For this review, take the finished solid that the model builds, in its own axes (mm). Coordinates: 2 decimals unless noted, no trailing zeros. Loops run counter-clockwise (first coordinate to the right, second up) from the corner with the lowest first, then second, coordinate; pieces in that order, holes last. Notation, with made-up numbers: (-15, -38.75) - (30, -38.75) arc R14 ccw to (30, -12.75) - close; hole circle Ø4 at (22.25, 3.25). An arc over 180 degrees is marked (long way). Use one line per item in the form item = value. Start each with the question number.
1. To check wall thickness, follow probe 1 along Y at (x, z) = (73.25, -4.5); probe 2 along Z at (x, y) = (-114, 27.5); probe 3 along Y at (x, z) = (-128.5, -1.75). State the ranges of each line that lie inside material, in increasing order.
2. Add section C-C on y = 38.5. Give the boundary of the cut face in (x, z), and give its area (3 significant figures).
3. Add section A-A on z = -1.5. Give the boundary of the cut face in (x, y), and give its area (3 significant figures).
4. Add section B-B on x = 83.5. Give the boundary of the cut face in (y, z), and give its area (3 significant figures).
5. Add section D-D on x = -32. Give the boundary of the cut face in (y, z).
6. For pin 1 Ø0.9 at (x, y) = (-120.5, -49) entering from +Z; pin 2 Ø3 at (x, z) = (-115.5, -0.5) entering from -Y; pin 3 Ø3 at (y, z) = (68.08, -4.5) entering from -X; pin 4 Ø4 at (x, z) = (-121.5, -3) entering from -Y, all flat-tipped, find the tip position at first contact; note any pin that passes through.
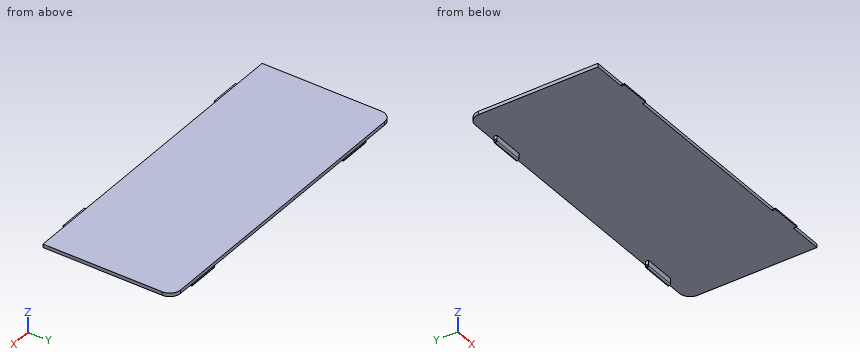
```python
from build123d import *

# Parameters (mm, degrees)
EXTRUDE_1_DEPTH     = 3.2
SKETCH_2_W          = 28
SKETCH_2_H          = 3
CUT_EXTRUDE_1_DEPTH = 2
SKETCH_3_W          = 29
SKETCH_3_H          = 2.8
EXTRUDE_2_DEPTH     = 6.5
SKETCH_4_R          = 1
CUT_EXTRUDE_2_DEPTH = 270.771576627
FILLET_1_R          = 1.5


with BuildPart() as part:
    # 草图1 → 凸台-拉伸1 (new body)
    with BuildSketch(Plane.XY):
        with BuildLine():
            Line((-107.202531646, -47.623114492), (64.797468354, -47.623114492))
            Line((64.797468354, -47.623114492), (64.797468354, -50.623114492))
            Line((64.797468354, -50.623114492), (92.797468354, -50.623114492))
            Line((92.797468354, -50.623114492), (92.797468354, -47.623114492))
            Line((92.797468354, -47.623114492), (123.797468354, -47.623114492))
            Line((123.797468354, -47.623114492), (123.797468354, 62.376885508))
            ThreePointArc((123.797468354, 62.376885508), (120.868536166, 69.447953319), (113.797468354, 72.376885508))
            Line((113.797468354, 72.376885508), (-156.202531646, 72.376885508))
            ThreePointArc((-156.202531646, 72.376885508), (-163.273599457, 69.447953319), (-166.202531646, 62.376885508))
            Line((-166.202531646, 62.376885508), (-166.202531646, -47.623114492))
            Line((-166.202531646, -47.623114492), (-135.202531646, -47.623114492))
            Line((-135.202531646, -47.623114492), (-135.202531646, -50.623114492))
            Line((-135.202531646, -50.623114492), (-107.202531646, -50.623114492))
            Line((-107.202531646, -50.623114492), (-107.202531646, -47.623114492))
        make_face()
    extrude(amount=EXTRUDE_1_DEPTH)

    # 草图2 → 切除-拉伸1 (cut)
    with BuildSketch(Plane.XY.offset(3.2)):
        with Locations((-121.202531646, -49.123114492)):
            Rectangle(SKETCH_2_W, SKETCH_2_H)
        with Locations((78.797468354, -49.123114492)):
            Rectangle(SKETCH_2_W, SKETCH_2_H)
    extrude(amount=-CUT_EXTRUDE_1_DEPTH, mode=Mode.SUBTRACT)

    # 草图3 → 凸台-拉伸2 (add)
    with BuildSketch(Plane.XY):
        with Locations((-121.502531646, 67.976885508)):
            Rectangle(SKETCH_3_W, SKETCH_3_H)
        with Locations((79.097468354, 67.976885508)):
            Rectangle(SKETCH_3_W, SKETCH_3_H)
    extrude(amount=-EXTRUDE_2_DEPTH)

    # 草图4 → 切除-拉伸2 (cut, through all)
    with BuildSketch(Plane(origin=(93.597468354, 0, 0), x_dir=(0, 0, -1), z_dir=(1, 0, 0))):
        with Locations((4.5, 68.076885508)):
            Circle(SKETCH_4_R)
    extrude(amount=-CUT_EXTRUDE_2_DEPTH, mode=Mode.SUBTRACT)

    # 圆角1
    # the kernel refuses this fillet: 1.5 mm, written as the material it takes off along each edge
    with BuildSketch(Plane(origin=(60.847468354, 66.576885508, -6.5), x_dir=(0, 0, 1), z_dir=(1, 0, 0)), Plane(origin=(97.347468354, 69.376885508, -6.5), x_dir=(0, 0, 1), z_dir=(-1, 0, 0))) as fillet_1_piece_1:
        with BuildLine():
            CenterArc((FILLET_1_R, -FILLET_1_R), FILLET_1_R, 90, 90)
            Line((0, -FILLET_1_R), (0, 0))
            Line((0, 0), (FILLET_1_R, 0))
        make_face()
    extrude(amount=36.5, mode=Mode.SUBTRACT)
    with BuildSketch(Plane(origin=(-103.252531646, 66.576885508, -6.5), x_dir=(0, 0, 1), z_dir=(-1, 0, 0)), Plane(origin=(-139.752531646, 69.376885508, -6.5), x_dir=(0, 0, 1), z_dir=(1, 0, 0))) as fillet_1_piece_2:
        with BuildLine():
            CenterArc((FILLET_1_R, FILLET_1_R), FILLET_1_R, 180, 90)
            Line((0, FILLET_1_R), (0, 0))
            Line((0, 0), (FILLET_1_R, 0))
        make_face()
    extrude(amount=36.5, mode=Mode.SUBTRACT)


solid = part.part
```
Conclusion:
q1.probe_1 = 66.58 to 67.08, 69.08 to 69.38
q1.probe_2 = 0 to 3.2
q1.probe_3 = 66.58 to 69.38
q2.outline = (-166.2, 0) - (123.8, 0) - (123.8, 3.2) - (-166.2, 3.2) - close
q2.area = 928 mm^2
q3.outline = (-136, 66.58) - (-107, 66.58) - (-107, 69.38) - (-136, 69.38) - close; (64.6, 66.58) - (93.6, 66.58) - (93.6, 69.38) - (64.6, 69.38) - close
q3.area = 162 mm^2
q4.outline = (-50.62, 0) - (66.58, 0) - (66.58, -5) arc R1.5 ccw to (67.98, -6.5) arc R1.5 ccw to (69.38, -5) - (69.38, 0) - (72.38, 0) - (72.38, 3.2) - (-47.62, 3.2) - (-47.62, 1.2) - (-50.62, 1.2) - close; hole circle Ø2 at (68.08, -4.5)
q4.area = 402 mm^2
q5.outline = (-47.62, 0) - (72.38, 0) - (72.38, 3.2) - (-47.62, 3.2) - close
q6.pin_1 = 1.2
q6.pin_2 = -50.62
q6.pin_3 = -136
q6.pin_4 = 66.58
